from build123d import *

# Parameters (mm, degrees)
F0_R     = 11.2
F1_DEPTH = 7
F2_R     = 1.5


with BuildPart() as f1:
    # F0 (on Top) → F1 (new body)
    with BuildSketch(Plane.XY):
        Polygon((-4.691563, 38.529854), (-14.480257, 9.15993), (-37.200133, -12.627188), (-31.022051, -23.32794), (-0.692603, -17.120235), (29.535532, -25.902666), (35.713614, -15.201914), (15.17286, 7.960306), (7.664601, 38.529854), align=None)
        Circle(F0_R, mode=Mode.SUBTRACT)
    extrude(amount=F1_DEPTH)

    # F2
    f2_edges = [f1.edges().sort_by_distance(p)[0] for p in [
        (-9.58591, 23.844892, 7),
        (-25.840195, -1.733629, 7),
        (-34.111092, -17.977564, 7),
        (14.421464, -21.511451, 7),
        (32.624573, -20.55229, 7),
        (25.443237, -3.620804, 7),
        (11.418731, 23.24508, 7),
        (1.486519, 38.529854, 7),
        (-15.857327, -20.224088, 7),
        (-11.2, 0, 7),
        (15.17286, 7.960306, 3.5),
        (7.664601, 38.529854, 3.5),
        (11.418731, 23.24508, 0),
        (14.421464, -21.511451, 0),
        (32.624573, -20.55229, 0),
        (25.443237, -3.620804, 0),
        (1.486519, 38.529854, 0),
        (-9.58591, 23.844892, 0),
        (-25.840195, -1.733629, 0),
        (-34.111092, -17.977564, 0),
        (-15.857327, -20.224088, 0),
        (-11.2, 0, 0),
    ]]
    fillet(f2_edges, radius=F2_R)


solid = f1.part
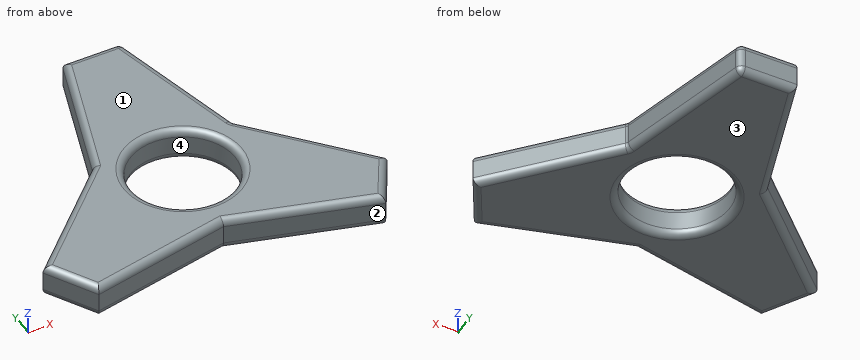
For this review, take the finished solid that the model builds, in its own axes (mm). Face numbers are marked on the shaded views. A direction names the side the tool comes from. Round coordinates to 2 decimals unless told otherwise and drop trailing zeros. Write each loop counter-clockwise with the first axis right and the second up, starting at its lowest first coordinate (ties: lowest second). Pieces come first, ordered by that corner, then holes. Notation, with made-up numbers: (-27.75, 48) - (13.25, 48) arc R19 ccw to (13.25, 83) - close; hole circle Ø11 at (53.5, 48). An arc over 180 degrees is marked (long way). Use a Markdown table: item, result.
Q1. Machinability: for the marked faces 1 and 2, which of the approach directions +Z, -Z, +X, -X, +Y, -Y give a long, thin tool a straight path to every point of the face, cutting with its end or side? Answer none if there is none.
Derived:
| item | result |
|---|---|
| face 1 | +Z, +X, -X, +Y, -Y |
| face 2 | +Z, -Z, -Y |
Q2. Wall thickness on line 1 along Y through (x, z) = (0, 2.95); line 2 along Y through (x, z) = (-0.5, 0.5); line 3 along X through (y, z) = (4.5, 1): over which ranges is each line inside the solid? List them lowest first.
Derived:
| item | result |
|---|---|
| line 1 | y = -17.32 to -11.2, 11.2 to 38.53 |
| line 2 | y = -16.78 to -11.57, 11.57 to 38.15 |
| line 3 | x = -19.22 to -10.35, 10.35 to 18.13 |
Q3. We need section A-A (z = 4). Give the boundary of the cut face in (x, y).
Derived:
| item | result |
|---|---|
| outline | (-37.2, -12.63) - (-31.02, -23.33) - (-0.69, -17.12) - (29.54, -25.9) - (35.71, -15.2) - (15.42, 7.68) arc R1.5 cw to (15.08, 8.32) - (7.95, 37.39) arc R1.5 ccw to (6.49, 38.53) - (-4.69, 38.53) - (-14.48, 9.16) - close; hole circle Ø22.4 at (0, 0) |
Q4. The part is to be moulded in two halves that separate along X. For the marked faces 3 and 4, say which applies: pulls with the +X half, pulls with the -X half, needs draft (parallel to the pull), parting line crosses it, or undercut.
Derived:
| item | result |
|---|---|
| face 3 | needs draft |
| face 4 | undercut |
Q5. Clearance check with flat-ended pins moving along their axes: pin 1 (2 mm diameter, centred on x = -19.5, z = 3, fed in from -Y); pin 2 (1 mm diameter, centred on y = 10.5, z = 1.5, fed in from +X); pin 3 (2 mm diameter, centred on x = -29, y = -4.5, fed in from -Z). State where each tip first meets the part, or that it passes through.
Derived:
| item | result |
|---|---|
| pin 1 | stops at y = -21.17 |
| pin 2 | stops at x = 14.67 |
| pin 3 | stops at z = 0.17 |
